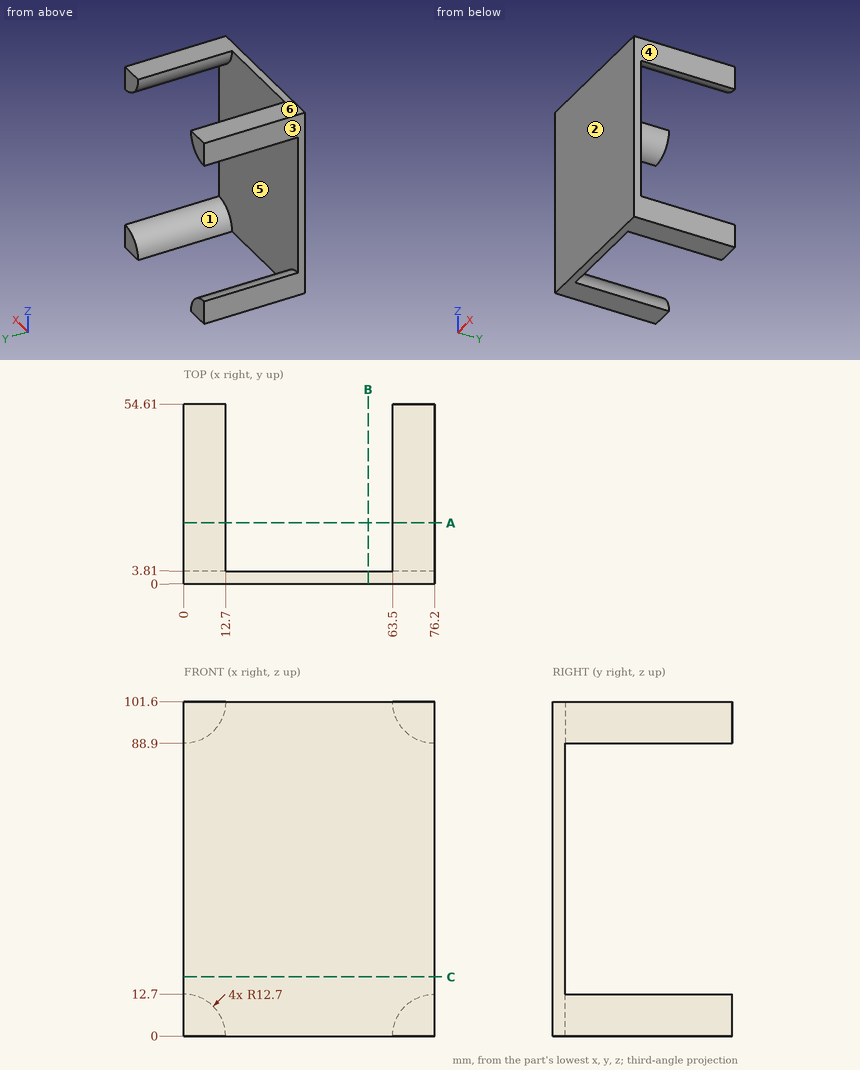
Geometry check sheet. Reference: drawing and pictorial views, mm from the part's lowest x, y, z. A direction names the side the tool comes from. Coordinates: 2 decimals unless noted, no trailing zeros. Loops run counter-clockwise (first coordinate to the right, second up) from the corner with the lowest first, then second, coordinate; pieces in that order, holes last.
1) Access from +Z, -Z, +X, -X, +Y, -Y to the whole of each face (thin tool, end or side, straight path). Record for the marked faces 1 and 2.
2) Sectioned sample at C-C (z = 18). Record the boundary of the cut face in (x, y), and give its area (3 significant figures).
3) Sectioned sample at B-B (x = 56). Record the boundary of the cut face in (y, z).
4) Sectioned sample at A-A (y = 18.5). Count the separate pieces of the cut face and the enclosed holes in it, and give its area (3 significant figures).
5) Gauge pin test, flat ends, axial feed: pin 1 (12 mm diameter, centred on x = 20, y = 37.5, fed in from -Z); pin 2 (8 mm diameter, centred on x = 31, z = 61.5, fed in from +Y). Record the tip position at first contact, or that the pin passes through.
6) Material ranges on probe 1 along Y at (x, z) = (33.5, 43); probe 2 along X at (y, z) = (51.5, 91) (3 decimals); probe 3 along X at (y, z) = (43, 11), recorded low to high.
7) Release check for a two-part mould opening along X. For the marked faces 3, 4, 5 and 6 record: released by +X, released by -X, zero draft, split by the parting line, or undercut.
Check sheet entries:
1. face 1: +Y
1. face 2: +Z, -Z, +X, -X, -Y
2. outline: (0, 0) - (76.2, 0) - (76.2, 3.81) - (0, 3.81) - close
2. area: 290 mm2
3. outline: (0, 0) - (3.81, 0) - (3.81, 101.6) - (0, 101.6) - close
4. separate pieces: 4
4. enclosed holes: 0
4. area: 507 mm2
5. pin 1: passes through
5. pin 2: stops at y = 3.81
6. probe 1: y = 0 to 3.81
6. probe 2: x = 0 to 6.995, 69.205 to 76.2
6. probe 3: x = 0 to 6.35, 69.85 to 76.2
7. face 3: released by -X
7. face 4: released by +X
7. face 5: undercut
7. face 6: zero draft
